Source: three-view drawing plus pictorial views. Frame: mm from the lowest corner of the part. Give positions to 0.01 mm unless a question says otherwise; leave off trailing zeros. Loops run counter-clockwise (first coordinate to the right, second up) from the corner with the lowest first, then second, coordinate; pieces in that order, holes last.
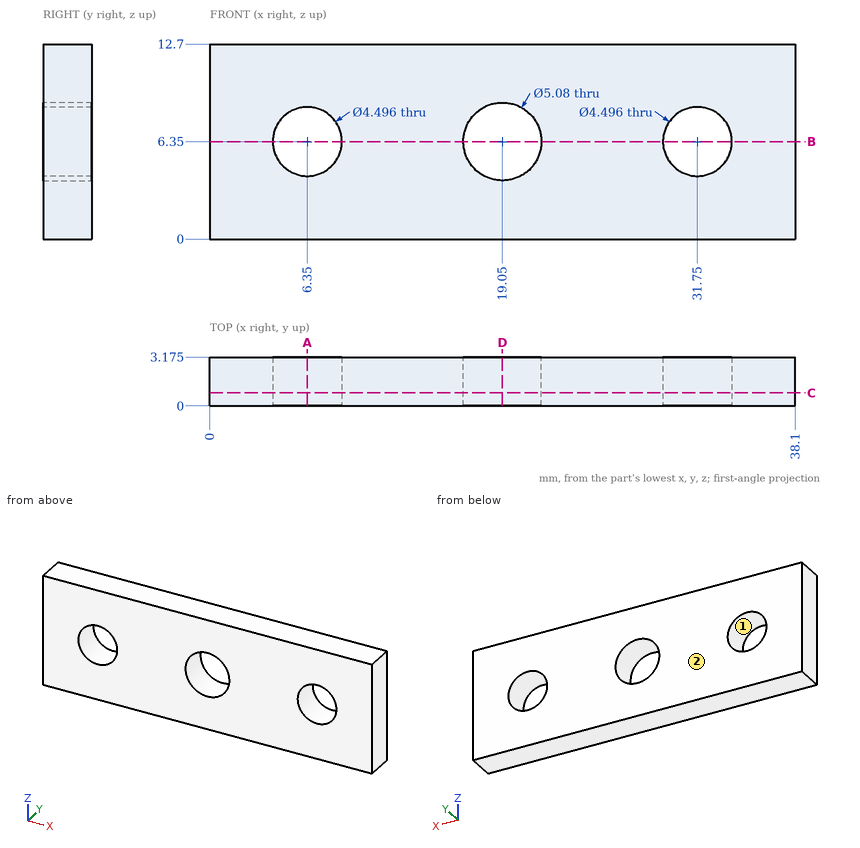
1) Pull-direction query (X, two-part tool) for the marked faces 1 and 2; classes: released by +X, released by -X, zero draft, split by the parting line, or undercut.
Checks:
face 1: undercut
face 2: zero draft
2) Cut plane D-D (x = 19.05). Return loops of the section in (y, z) (3 decimals).
Checks:
outline: (0, 0) - (3.175, 0) - (3.175, 3.81) - (0, 3.81) - close; (0, 8.89) - (3.175, 8.89) - (3.175, 12.7) - (0, 12.7) - close
3) Cut plane C-C (y = 0.85). Return loops of the section in (x, z), and give its area (3 significant figures).
Checks:
outline: (0, 0) - (38.1, 0) - (38.1, 12.7) - (0, 12.7) - close; hole circle Ø4.5 at (6.35, 6.35); hole circle Ø5.08 at (19.05, 6.35); hole circle Ø4.5 at (31.75, 6.35)
area: 432 mm2
4) Ray query, probe 1 along X at (y, z) = (0.65, 6.25); probe 2 along Z at (x, y) = (6.35, 1.6); probe 3 along X at (y, z) = (0.4, 7.25) (1 decimal). Return the intervals inside material, ascending.
Checks:
probe 1: x = 0 to 4.1, 8.6 to 16.51, 21.59 to 29.5, 34 to 38.1
probe 2: z = 0 to 4.1, 8.6 to 12.7
probe 3: x = 0 to 4.3, 8.4 to 16.7, 21.4 to 29.7, 33.8 to 38.1
5) Cut plane B-B (z = 6.35). Return loops of the section in (x, y) (1 decimal).
Checks:
outline: (0, 0) - (4.1, 0) - (4.1, 3.2) - (0, 3.2) - close; (8.6, 0) - (16.5, 0) - (16.5, 3.2) - (8.6, 3.2) - close; (21.6, 0) - (29.5, 0) - (29.5, 3.2) - (21.6, 3.2) - close; (34, 0) - (38.1, 0) - (38.1, 3.2) - (34, 3.2) - close
6) Cut plane A-A (x = 6.35). Return loops of the section in (y, z) (1 decimal).
Checks:
outline: (0, 0) - (3.2, 0) - (3.2, 4.1) - (0, 4.1) - close; (0, 8.6) - (3.2, 8.6) - (3.2, 12.7) - (0, 12.7) - close
